Source: CAD feature listing. Evaluate the final solid. Frame: model axes, mm. Face numbers are marked on the shaded views. A direction names the side the tool comes from. Give positions to 0.01 mm unless a question says otherwise; leave off trailing zeros. Write each loop counter-clockwise with the first axis right and the second up, starting at its lowest first coordinate (ties: lowest second). Pieces come first, ordered by that corner, then holes. Notation, with made-up numbers: (66.25, -15.5) - (115.25, -15.5) arc R17 ccw to (115.25, 16.5) - close; hole circle Ø9 at (37, 86). An arc over 180 degrees is marked (long way). Answer as a JSON object with one key per item and string values. Group by question number.
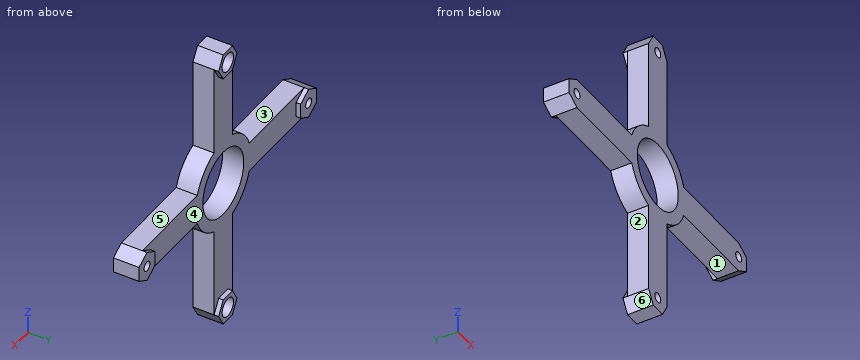
from build123d import *

# Parameters (mm, degrees)
SKETCH1_R           = 11.125
SKETCH1_R_2         = 1.6
BOSS_EXTRUDE1_DEPTH = 7
SKETCH3_R           = 3.1
CUT_EXTRUDE1_DEPTH  = 2.8
SKETCH2_R           = 1.6
SKETCH2_R_2         = 3.1
BOSS_EXTRUDE2_DEPTH = 1.5


with BuildPart() as part:
    # Sketch1 → Boss-Extrude1 (new body)
    with BuildSketch(Plane(origin=(0, 0, 0), x_dir=(1, 0, 0), z_dir=(0, 1, 0))):
        with BuildLine():
            Line((44, 5), (48.330127019, 2.5))
            Line((48.330127019, 2.5), (48.330127019, -2.5))
            Line((48.330127019, -2.5), (44, -5))
            Line((44, -5), (14.142135624, -5))
            ThreePointArc((14.142135624, -5), (10.606601718, -10.606601718), (5, -14.142135624))
            Line((5, -14.142135624), (5, -44))
            Line((5, -44), (2.5, -48.330127019))
            Line((2.5, -48.330127019), (-2.5, -48.330127019))
            Line((-2.5, -48.330127019), (-5, -44))
            Line((-5, -44), (-5, -14.142135624))
            ThreePointArc((-5, -14.142135624), (-10.606601718, -10.606601718), (-14.142135624, -5))
            Line((-14.142135624, -5), (-44, -5))
            Line((-44, -5), (-48.330127019, -2.5))
            Line((-48.330127019, -2.5), (-48.330127019, 2.5))
            Line((-48.330127019, 2.5), (-44, 5))
            Line((-44, 5), (-14.142135624, 5))
            ThreePointArc((-14.142135624, 5), (-10.606601718, 10.606601718), (-5, 14.142135624))
            Line((-5, 14.142135624), (-5, 44))
            Line((-5, 44), (-2.5, 48.330127019))
            Line((-2.5, 48.330127019), (2.5, 48.330127019))
            Line((2.5, 48.330127019), (5, 44))
            Line((5, 44), (5, 14.142135624))
            ThreePointArc((5, 14.142135624), (10.606601718, 10.606601718), (14.142135624, 5))
            Line((14.142135624, 5), (44, 5))
        make_face()
        with Locations(Location((0, 0, 0), (0, 0, 270))):
            Circle(SKETCH1_R, mode=Mode.SUBTRACT)
        with Locations(Location((44, 0, 0), (0, 0, 270))):
            Circle(SKETCH1_R_2, mode=Mode.SUBTRACT)
        with Locations(Location((0, 44, 0), (0, 0, 270))):
            Circle(SKETCH1_R_2, mode=Mode.SUBTRACT)
        with Locations(Location((-44, 0, 0), (0, 0, 270))):
            Circle(SKETCH1_R_2, mode=Mode.SUBTRACT)
        with Locations(Location((0, -44, 0), (0, 0, 270))):
            Circle(SKETCH1_R_2, mode=Mode.SUBTRACT)
    extrude(amount=BOSS_EXTRUDE1_DEPTH)

    # Sketch3 → Cut-Extrude1 (cut)
    with BuildSketch(Plane(origin=(0, 7, 0), x_dir=(1, 0, 0), z_dir=(0, 1, 0))):
        with Locations(Location((0, 44, 0), (0, 0, 270))):
            Circle(SKETCH3_R)
        with Locations(Location((0, -44, 0), (0, 0, 270))):
            Circle(SKETCH3_R)
    extrude(amount=-CUT_EXTRUDE1_DEPTH, mode=Mode.SUBTRACT)

    # Sketch2 → Boss-Extrude2 (add)
    # profile 1 of 4: a face of its own
    with BuildSketch(Plane(origin=(0, 7, 0), x_dir=(1, 0, 0), z_dir=(0, 1, 0))):
        Polygon((-44, 5), (-48.330127019, 2.5), (-48.330127019, -2.5), (-44, -5), (-39.669872981, -2.5), (-39.669872981, 2.5), align=None)
        with Locations(Location((-44, 0, 0), (0, 0, 270))):
            Circle(SKETCH2_R, mode=Mode.SUBTRACT)
    # profile 2 of 4: a face of its own
    with BuildSketch(Plane(origin=(0, 7, 0), x_dir=(1, 0, 0), z_dir=(0, 1, 0))):
        Polygon((48.330127019, 2.5), (44, 5), (39.669872981, 2.5), (39.669872981, -2.5), (44, -5), (48.330127019, -2.5), align=None)
        with Locations(Location((44, 0, 0), (0, 0, 270))):
            Circle(SKETCH2_R, mode=Mode.SUBTRACT)
    # profile 3 of 4: a face of its own
    with BuildSketch(Plane(origin=(0, 7, 0), x_dir=(1, 0, 0), z_dir=(0, 1, 0))):
        Polygon((2.5, 48.330127019), (-2.5, 48.330127019), (-5, 44), (-2.5, 39.669872981), (2.5, 39.669872981), (5, 44), align=None)
        with Locations(Location((0, 44, 0), (0, 0, 270))):
            Circle(SKETCH2_R_2, mode=Mode.SUBTRACT)
    # profile 4 of 4: a face of its own
    with BuildSketch(Plane(origin=(0, 7, 0), x_dir=(1, 0, 0), z_dir=(0, 1, 0))):
        Polygon((-2.5, -48.330127019), (2.5, -48.330127019), (5, -44), (2.5, -39.669872981), (-2.5, -39.669872981), (-5, -44), align=None)
        with Locations(Location((0, -44, 0), (0, 0, 270))):
            Circle(SKETCH2_R_2, mode=Mode.SUBTRACT)
    extrude(amount=BOSS_EXTRUDE2_DEPTH)


solid = part.part
Q1. Reachability of the marked faces 1, 2 and 3 from +Z, -Z, +X, -X, +Y, -Y: full face, straight path, thin tool, end or side. Return the list, or none.
Q2. Section B-B on z = 0. Return the cut outline in (x, y) (3 decimals), then the cut area to 3 significant figures.
Q3. Section D-D on x = -23. Return the cut outline in (y, z).
Q4. Draft query along Z for the marked faces 4, 5 and 6. Return one class per face: released by +Z, released by -Z, zero draft, split by the parting line, or undercut.
Q5. Section C-C on y = 3. State how many separate pieces and enclosed holes the cut face has, then the cut area to 3 significant figures.
Q6. Ray query, probe 1 along X at (y, z) = (6, 0) (3 decimals); probe 2 along X at (y, z) = (7.2, 44); probe 3 along Z at (x, y) = (-22, 3). Return the intervals inside material, ascending. Write a range as [from, to].
Q7. Section A-A on x = 0. Return the cut outline in (y, z) (3 decimals), then the cut area to 3 significant figures.
Q8. First-contact query: pin 1 Ø4 at (x, y) = (5.5, 5) entering from +Z; pin 2 Ø5.5 at (x, z) = (0, 44) entering from +Y; pin 3 Ø1 at (x, z) = (-2, 26.5) entering from +Y. Flat tips, straight axial feed; report the tip coordinate or a pass-through.
Taken from the geometry:
{
 "1": {"face 1": "-Z, +X, +Y, -Y", "face 2": "-Z, -X, +Y, -Y", "face 3": "+Z, -X, +Y, -Y"},
 "2": {"outline": "(-48.33, 0) - (-45.6, 0) - (-45.6, 8.5) - (-48.33, 8.5) - close; (-42.4, 0) - (-11.125, 0) - (-11.125, 7) - (-39.67, 7) - (-39.67, 8.5) - (-42.4, 8.5) - close; (11.125, 0) - (42.4, 0) - (42.4, 8.5) - (39.67, 8.5) - (39.67, 7) - (11.125, 7) - close; (45.6, 0) - (48.33, 0) - (48.33, 8.5) - (45.6, 8.5) - close", "area": "492 mm²"},
 "3": {"outline": "(0, -5) - (7, -5) - (7, 5) - (0, 5) - close"},
 "4": {"face 4": "undercut", "face 5": "released by +Z", "face 6": "released by -Z"},
 "5": {"separate pieces": "1", "enclosed holes": "5", "area": "1,590 mm²"},
 "6": {"probe 1": "x = [-48.33, -45.6], [-42.4, -11.125], [11.125, 42.4], [45.6, 48.33]", "probe 2": "x = [-5, -3.1], [3.1, 5]", "probe 3": "z = [-5, 5]"},
 "7": {"outline": "(0, -48.33) - (8.5, -48.33) - (8.5, -47.1) - (4.2, -47.1) - (4.2, -45.6) - (0, -45.6) - close; (0, -42.4) - (4.2, -42.4) - (4.2, -40.9) - (8.5, -40.9) - (8.5, -39.67) - (7, -39.67) - (7, -11.125) - (0, -11.125) - close; (0, 11.125) - (7, 11.125) - (7, 39.67) - (8.5, 39.67) - (8.5, 40.9) - (4.2, 40.9) - (4.2, 42.4) - (0, 42.4) - close; (0, 45.6) - (4.2, 45.6) - (4.2, 47.1) - (8.5, 47.1) - (8.5, 48.33) - (0, 48.33) - close", "area": "467 mm²"},
 "8": {"pin 1": "stops at z = 46.6", "pin 2": "stops at y = 4.2", "pin 3": "stops at y = 7"}
}
